```python
from build123d import *

# Parameters (mm, degrees)
SKETCH_1_W          = 136.3
SKETCH_1_H          = 136.3
EXTRUDE_1_DEPTH     = 4
EXTRUDE_2_DEPTH     = 100
CUT_EXTRUDE_1_DEPTH = 100
SKETCH_4_W          = 60.5
SKETCH_4_H          = 100
EXTRUDE_3_DEPTH     = 60.5


with BuildPart() as part:
    # 草图1 → 凸台-拉伸1 (new body)
    with BuildSketch(Plane(origin=(0, 0, 0), x_dir=(1, 0, 0), z_dir=(0, 1, 0))):
        Rectangle(SKETCH_1_W, SKETCH_1_H)
    extrude(amount=EXTRUDE_1_DEPTH)

    # 草图2 → 凸台-拉伸2 (add)
    with BuildSketch(Plane(origin=(0, 4, 0), x_dir=(1, 0, 0), z_dir=(0, 1, 0))):
        Polygon((30.25, 30.25), (-30.25, 30.25), (-30.25, -30.25), (30.25, -30.25), (30.25, -33.35), (-33.35, -33.35), (-33.35, -1.55), (-63.85, -1.55), (-63.85, 1.55), (-33.35, 1.55), (-33.35, 33.35), (30.25, 33.35), align=None)
    extrude(amount=EXTRUDE_2_DEPTH)

    # 草图3 → 切除-拉伸1 (cut)
    with BuildSketch(Plane.XY.offset(1.55)):
        Polygon((-63.85, 4), (-33.35, 72), (-33.35, 104), (-63.85, 104), align=None)
    extrude(amount=-CUT_EXTRUDE_1_DEPTH, mode=Mode.SUBTRACT)

    # 草图4 → 凸台-拉伸3 (add)
    with BuildSketch(Plane(origin=(-30.25, 0, 0), x_dir=(0, 0, -1), z_dir=(1, 0, 0))):
        with Locations((0, 54)):
            Rectangle(SKETCH_4_W, SKETCH_4_H)
    extrude(amount=EXTRUDE_3_DEPTH)


solid = part.part
```
The model under review builds one solid part; all positions refer to its coordinate system, in mm. A direction names the side the tool comes from. Round coordinates to 2 decimals unless told otherwise and drop trailing zeros. Write each loop counter-clockwise with the first axis right and the second up, starting at its lowest first coordinate (ties: lowest second). Pieces come first, ordered by that corner, then holes. Notation, with made-up numbers: (-21, -20.75) -> (15, -20.75) arc R20 ccw to (15, -13.75) -> close; hole circle Ø5 at (10.25, 67.25). An arc over 180 degrees is marked (long way). Use CSV: the item, a comma, the result in double quotes.
Q1. For pin 1 Ø19 at (x, y) = (-7.5, 74.5) entering from +Z; pin 2 Ø1.5 at (y, z) = (29, 34) entering from -X; pin 3 Ø12 at (x, z) = (-54, 32.5) entering from -Y; pin 4 Ø2 at (x, z) = (-38, 28.5) entering from +Y, all flat-tipped, find the tip position at first contact; note any pin that passes through.
Checks:
pin 1,"z = 33.35"
pin 2,"x = -33.35"
pin 3,"y = 0"
pin 4,"y = 4"
Q2. Consider section B-B (x = 12.5). Give the boundary of the cut face in (y, z).
Checks:
outline,"(0, -68.15) -> (4, -68.15) -> (4, -33.35) -> (104, -33.35) -> (104, 33.35) -> (4, 33.35) -> (4, 68.15) -> (0, 68.15) -> close"
Q3. Consider section A-A (z = 25). Give the boundary of the cut face in (x, y), then the cut area to 3 significant figures.
Checks:
outline,"(-68.15, 0) -> (68.15, 0) -> (68.15, 4) -> (30.25, 4) -> (30.25, 104) -> (-33.35, 104) -> (-33.35, 4) -> (-68.15, 4) -> close"
area,"6,910 mm²"
Q4. Consider section C-C (y = 90.5). Give the boundary of the cut face in (x, z).
Checks:
outline,"(-33.35, -33.35) -> (30.25, -33.35) -> (30.25, 33.35) -> (-33.35, 33.35) -> close"
Q5. Consider section D-D (x = 56.5). Give the boundary of the cut face in (y, z).
Checks:
outline,"(0, -68.15) -> (4, -68.15) -> (4, 68.15) -> (0, 68.15) -> close"
Q6. For faces 1 (the flat face through (-2, 53, -33.35)), 2 (the flat face through (-1, 53, 33.35)), 3 (the flat face through (-33.35, 53, 8)), 4 (the flat face through (-45, 30, 1.55)), 5 (the flat face through (-42, 22, -1.55)), list the 3-axis set-ups (+Z, -Z, +X, -X, +Y, -Y) from which the entire face can be reached by the end or side of a thin tool; tool diameter is ignored.
Checks:
face 1,"-Z, +X, -X, +Y"
face 2,"+Z, +X, -X, +Y"
face 3,"-X, +Y"
face 4,"+Z, -X, +Y"
face 5,"-Z, -X, +Y"
Q7. To check wall thickness, follow probe 1 along Z at (x, y) = (-21, 69); probe 2 along Y at (x, z) = (-26, 55); probe 3 along X at (y, z) = (98, 26). State the ranges of each line that lie inside material, in increasing order. Write a range as [from, to].
Checks:
probe 1,"[-33.35, 33.35]"
probe 2,"[0, 4]"
probe 3,"[-33.35, 30.25]"
